Geometry check sheet. Reference: the model listing, model coordinates, mm. Face numbers are marked on the shaded views. A direction names the side the tool comes from. Coordinates: 2 decimals unless noted, no trailing zeros. Loops run counter-clockwise (first coordinate to the right, second up) from the corner with the lowest first, then second, coordinate; pieces in that order, holes last. Notation, with made-up numbers: (-17.5, 76.5) - (8.5, 76.5) arc R24 cw to (8.5, 94.5) - close; hole circle Ø9 at (19.5, 35.25). An arc over 180 degrees is marked (long way). Write item = value, one per line. Start each with the question number.
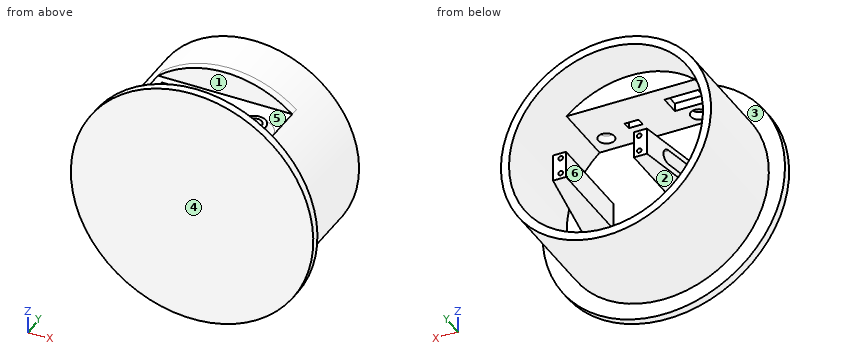
from build123d import *

# Parameters (mm, degrees)
SKETCH4_R                   = 65
SKETCH4_R_2                 = 60
EXTRUDE_THIN1_DEPTH         = 75
SKETCH5_R                   = 75
BOSS_EXTRUDE1_DEPTH         = 5
BOSS_EXTRUDE2_START         = -40
SKETCH6_W                   = 83.06623863
SKETCH6_H                   = 5
BOSS_EXTRUDE2_DEPTH         = 40
CUT_EXTRUDE1_START          = -40
CUT_EXTRUDE1_DEPTH          = 35
SKETCH8_W                   = 7.6
SKETCH8_H                   = 16.75
BOSS_EXTRUDE3_DEPTH         = 57.3
CHAMFER1_SIZE               = 10
CHAMFER1_SIZE_2             = 60
M3_5X0_6_TAPPED_HOLE1_D     = 2.9
M3_5X0_6_TAPPED_HOLE1_DEPTH = 9.128752102
M3_5X0_6_TAPPED_HOLE1_TIP   = 0.871247898
CUT_EXTRUDE2_START          = -57.3
SKETCH11_W                  = 18.622960368
SKETCH11_H                  = 9.279079534
CUT_EXTRUDE2_DEPTH          = 42.3
FILLET1_R                   = 5
CUT_EXTRUDE3_REACH          = 165.936
SKETCH12_R                  = 5.1
SKETCH12_W                  = 20.8
SKETCH12_H                  = 12.6
SKETCH12_W_2                = 8.6
SKETCH12_H_2                = 5
SKETCH13_R                  = 7.5
SKETCH13_R_2                = 5
BOSS_EXTRUDE4_DEPTH         = 5
FILLET2_R                   = 4
CUT_EXTRUDE4_REACH          = 165.936
SKETCH14_R                  = 5


with BuildPart() as part:
    # Sketch4 → Extrude-Thin1 (new body)
    with BuildSketch(Plane(origin=(0, 0, 0), x_dir=(1, 0, 0), z_dir=(0, 1, 0))):
        Circle(SKETCH4_R)
        Circle(SKETCH4_R_2, mode=Mode.SUBTRACT)
    extrude(amount=EXTRUDE_THIN1_DEPTH)

    # Sketch5 → Boss-Extrude1 (add)
    with BuildSketch(Plane(origin=(0, 0, 0), x_dir=(1, 0, 0), z_dir=(0, 1, 0))):
        with Locations(Location((0, 0, 0), (0, 0, 270))):
            Circle(SKETCH5_R)
    extrude(amount=BOSS_EXTRUDE1_DEPTH)

    # Sketch6 → Boss-Extrude2 (add)
    with BuildSketch(Plane(origin=(0, 45, 0), x_dir=(1, 0, 0), z_dir=(0, 1, 0)).offset(BOSS_EXTRUDE2_START)):
        with Locations((0, -47.5)):
            Rectangle(SKETCH6_W, SKETCH6_H)
        with BuildLine():
            Line((41.533119315, -50), (0, -50))
            Line((0, -50), (0, -65))
            ThreePointArc((0, -65), (22.079402166, -61.135096303), (41.533119315, -50))
        make_face()
        with BuildLine():
            Line((0, -65), (0, -50))
            Line((0, -50), (-41.533119315, -50))
            ThreePointArc((-41.533119315, -50), (-22.079402166, -61.135096303), (0, -65))
        make_face()
        with BuildLine():
            Line((41.533119315, -50), (0, -50))
            Line((0, -50), (0, -65))
            ThreePointArc((0, -65), (22.079402166, -61.135096303), (41.533119315, -50))
        make_face()
        with BuildLine():
            Line((0, -65), (0, -50))
            Line((0, -50), (-41.533119315, -50))
            ThreePointArc((-41.533119315, -50), (-22.079402166, -61.135096303), (0, -65))
        make_face()
    extrude(amount=BOSS_EXTRUDE2_DEPTH)

    # Sketch7 → Cut-Extrude1 (cut)
    with BuildSketch(Plane(origin=(0, 45, 0), x_dir=(1, 0, 0), z_dir=(0, 1, 0)).offset(CUT_EXTRUDE1_START)):
        with BuildLine():
            Line((-41.533119315, -50), (41.533119315, -50))
            ThreePointArc((41.533119315, -50), (0, -65), (-41.533119315, -50))
        make_face()
    extrude(amount=CUT_EXTRUDE1_DEPTH, mode=Mode.SUBTRACT)

    # Sketch8 → Boss-Extrude3 (add)
    with BuildSketch(Plane(origin=(0, 5, 0), x_dir=(1, 0, 0), z_dir=(0, 1, 0))):
        with Locations((35, 0.125)):
            Rectangle(SKETCH8_W, SKETCH8_H)
        with Locations((-14.6, 0.125)):
            Rectangle(SKETCH8_W, SKETCH8_H)
    extrude(amount=BOSS_EXTRUDE3_DEPTH)

    # Chamfer1
    # the kernel refuses this chamfer: 60, 10 mm, written as the material it adds along each edge
    with BuildSketch(Plane(origin=(38.8, 5, -8.5), x_dir=(0.9750324932942595, -0.2220622368174739, 0), z_dir=(0, 0, 1))) as chamfer1_piece_1_section:
        Polygon((CHAMFER1_SIZE * 0.975032493294, CHAMFER1_SIZE * 0.222062236817), (-CHAMFER1_SIZE_2 * 0.222062236817, CHAMFER1_SIZE_2 * 0.975032493294), (0, 0), align=None)
    chamfer1_piece_1 = extrude(amount=16.75, mode=Mode.PRIVATE)
    chamfer1_piece_1 = split(chamfer1_piece_1, bisect_by=Plane(origin=(41.528502242, 62.3, -0.125), z_dir=(0, -1, 0)), keep=Keep.TOP, mode=Mode.PRIVATE)
    add(chamfer1_piece_1)
    with BuildSketch(Plane(origin=(-18.4, 5, -8.5), x_dir=(-0.9750324932942595, -0.2220622368174739, 0), z_dir=(0, 0, 1))) as chamfer1_piece_2_section:
        Polygon((CHAMFER1_SIZE * 0.975032493294, -CHAMFER1_SIZE * 0.222062236817), (-CHAMFER1_SIZE_2 * 0.222062236817, -CHAMFER1_SIZE_2 * 0.975032493294), (0, 0), align=None)
    chamfer1_piece_2 = extrude(amount=16.75, mode=Mode.PRIVATE)
    chamfer1_piece_2 = split(chamfer1_piece_2, bisect_by=Plane(origin=(-21.128502242, 62.3, -0.125), z_dir=(0, -1, 0)), keep=Keep.TOP, mode=Mode.PRIVATE)
    add(chamfer1_piece_2)

    # M3.5x0.6 Tapped Hole1
    with Locations(Plane(origin=(0, 62.3, 0), x_dir=(1, 0, 0), z_dir=(0, 1, 0))):
        with Locations((34.5, 4.95), (34.5, -4.95), (-14.1, 4.95), (-14.1, -4.95)):
            Hole(M3_5X0_6_TAPPED_HOLE1_D / 2, depth=M3_5X0_6_TAPPED_HOLE1_DEPTH)
            with Locations((0, 0, -(M3_5X0_6_TAPPED_HOLE1_DEPTH + M3_5X0_6_TAPPED_HOLE1_TIP / 2))):  # 118° drill point
                Cone(0, M3_5X0_6_TAPPED_HOLE1_D / 2, M3_5X0_6_TAPPED_HOLE1_TIP, mode=Mode.SUBTRACT)

    # Sketch11 → Cut-Extrude2 (cut)
    with BuildSketch(Plane(origin=(0, 62.3, 0), x_dir=(1, 0, 0), z_dir=(0, 1, 0)).offset(CUT_EXTRUDE2_START)):
        with Locations((-19.088519816, 0)):
            Rectangle(SKETCH11_W, SKETCH11_H)
    extrude(amount=CUT_EXTRUDE2_DEPTH, mode=Mode.SUBTRACT)

    # Fillet1
    # the kernel refuses this fillet: 5 mm, written as the material it adds along each edge
    with BuildSketch(Plane(origin=(-10.8, 47.3, -4.639539767), x_dir=(0, 0, 1), z_dir=(-1, 0, 0))) as fillet1_piece_1_section:
        with BuildLine():
            CenterArc((FILLET1_R, -FILLET1_R), FILLET1_R, 90, 90)
            Line((0, -FILLET1_R), (0, 0))
            Line((0, 0), (FILLET1_R, 0))
        make_face()
    fillet1_piece_1 = extrude(amount=23.05, mode=Mode.PRIVATE)
    fillet1_piece_1 = split(fillet1_piece_1, bisect_by=Plane(origin=(-21.396510454, 47.020937275, -3.518217567), z_dir=(0.9863939238321439, -0.1643989873053573, 0)), keep=Keep.TOP, mode=Mode.PRIVATE)
    add(fillet1_piece_1)
    with BuildSketch(Plane(origin=(-33.85, 47.3, 4.639539767), x_dir=(0, -1, 0), z_dir=(1, 0, 0))) as fillet1_piece_2_section:
        with BuildLine():
            CenterArc((FILLET1_R, FILLET1_R), FILLET1_R, 180, 90)
            Line((0, FILLET1_R), (0, 0))
            Line((0, 0), (FILLET1_R, 0))
        make_face()
    fillet1_piece_2 = extrude(amount=23.05, mode=Mode.PRIVATE)
    fillet1_piece_2 = split(fillet1_piece_2, bisect_by=Plane(origin=(-21.396510454, 47.020937275, 3.518217567), z_dir=(0.9863939238321439, -0.1643989873053573, 0)), keep=Keep.TOP, mode=Mode.PRIVATE)
    add(fillet1_piece_2)

    # Sketch12 → Cut-Extrude3 (cut, up to next)
    with BuildSketch(Plane.XY.offset(50), mode=Mode.PRIVATE) as cut_extrude3_sk1:
        with Locations((-26.133119315, 13.4)):
            Circle(SKETCH12_R)
    cut_extrude3_tool1 = extrude(cut_extrude3_sk1.sketch, amount=-CUT_EXTRUDE3_REACH, mode=Mode.PRIVATE) & part.part
    # Sketch12 → Cut-Extrude3 (cut, up to next)
    with BuildSketch(Plane.XY.offset(50), mode=Mode.PRIVATE) as cut_extrude3_sk2:
        with Locations((-26.133119315, 28.7)):
            Rectangle(SKETCH12_W, SKETCH12_H)
    cut_extrude3_tool2 = extrude(cut_extrude3_sk2.sketch, amount=-CUT_EXTRUDE3_REACH, mode=Mode.PRIVATE) & part.part
    # Sketch12 → Cut-Extrude3 (cut, up to next)
    with BuildSketch(Plane.XY.offset(50), mode=Mode.PRIVATE) as cut_extrude3_sk3:
        with Locations((10.2, 21.5)):
            Rectangle(SKETCH12_W_2, SKETCH12_H_2)
    cut_extrude3_tool3 = extrude(cut_extrude3_sk3.sketch, amount=-CUT_EXTRUDE3_REACH, mode=Mode.PRIVATE) & part.part
    add(cut_extrude3_tool1.solids().sort_by_distance((-26.133119, 13.4, 50))[0], mode=Mode.SUBTRACT)
    add(cut_extrude3_tool2.solids().sort_by_distance((-26.133119, 28.7, 50))[0], mode=Mode.SUBTRACT)
    add(cut_extrude3_tool3.solids().sort_by_distance((10.2, 21.5, 50))[0], mode=Mode.SUBTRACT)

    # Sketch13 → Boss-Extrude4 (add)
    with BuildSketch(Plane.XY.offset(50)):
        with Locations(Location((30.033119315, 15.715961892, 0), (0, 0, 180))):
            Circle(SKETCH13_R)
        with Locations((30.033119315, 15.715961892)):
            Circle(SKETCH13_R_2, mode=Mode.SUBTRACT)
    extrude(amount=BOSS_EXTRUDE4_DEPTH)

    # Fillet2
    # the kernel refuses this fillet: 4 mm, written as the material it adds along each edge
    with BuildSketch(Plane(origin=(30.033119315, 15.715961892, 50), x_dir=(-1, 0, 0), z_dir=(0, 1, 0))) as fillet2_piece_1:
        with BuildLine():
            CenterArc((7.5 + FILLET2_R, FILLET2_R), FILLET2_R, 180, 90)
            Line((7.5, FILLET2_R), (7.5, 0))
            Line((7.5, 0), (7.5 + FILLET2_R, 0))
        make_face()
    revolve(axis=Axis((30.033119315, 15.715961892, 50), (0, 0, 1)))

    # Sketch14 → Cut-Extrude4 (cut, up to next)
    with BuildSketch(Plane.XY.offset(50), mode=Mode.PRIVATE) as cut_extrude4_sk1:
        with Locations((30.033119315, 15.715961892)):
            Circle(SKETCH14_R)
    cut_extrude4_tool1 = extrude(cut_extrude4_sk1.sketch, amount=-CUT_EXTRUDE4_REACH, mode=Mode.PRIVATE) & part.part
    add(cut_extrude4_tool1.solids().sort_by_distance((30.033119, 15.715962, 50))[0], mode=Mode.SUBTRACT)


solid = part.part
(1) Draft check along Y on the marked faces 5, 6 and 7. Enter one of: pulls with the +Y half, pulls with the -Y half, needs draft (parallel to the pull), parting line crosses it, or undercut.
(2) Sectioned sample at C-C on x = 45. Enter the section's corners in (y, z), plus the area to 3 significant figures.
(3) Scan lines: line 1 (X direction, y = 12.5, z = -0.5); line 2 (X direction, y = 58, z = 4); line 3 (Z direction, x = -14.1, y = 56). Record each from-to range of solid material in increasing order.
(4) Sectioned sample at A-A on x = 0. Enter the section's corners in (y, z), plus the area to 4 significant figures.
(5) Sectioned sample at B-B on z = 30. Enter the section's corners in (x, y), plus the area to 3 significant figures.
(6) Depth check by flat-ended pin: pin 1 (5.5 mm diameter, centred on x = -23.5, y = 27, fed in from -Z); pin 2 (4 mm diameter, centred on y = 48, z = -35.5, fed in from -X); pin 3 (8 mm diameter, centred on y = 54.5, z = -50.5, fed in from +X). Enter the tip coordinate at first touch or a pass-through.
(7) Tool access check on the marked faces 1, 2, 3 and 4. Record the directions out of +Z, -Z, +X, -X, +Y, -Y that give a thin tool (end or side, any length) a straight path to the whole face; none if there is none.
Working result:
q1.face_5 = undercut
q1.face_6 = needs draft
q1.face_7 = pulls with the +Y half
q2.outline = (0, -60) - (5, -60) - (5, -46.9) - (75, -46.9) - (75, -39.69) - (5, -39.69) - (5, -8.5) - (27.8, -8.5) - (27.8, 8.25) - (5, 8.25) - (5, 39.69) - (75, 39.69) - (75, 46.9) - (5, 46.9) - (5, 60) - (0, 60) - close
q2.area = 1,990 mm2
q3.line_1 = -65 to -60, 31.2 to 47.55, 60 to 65
q3.line_2 = -64.88 to -59.87, -19.57 to -15.2, -13 to -10.8, 31.2 to 33.4, 35.6 to 39.97, 59.87 to 64.88
q3.line_3 = -63.45 to -58.32, -8.5 to -6.4, -3.5 to 3.5, 6.4 to 8.25, 58.32 to 63.45
q4.outline = (0, -75) - (5, -75) - (5, -65) - (75, -65) - (75, -60) - (5, -60) - (5, 45) - (45, 45) - (45, 60) - (75, 60) - (75, 65) - (40, 65) - (40, 50) - (5, 50) - (5, 75) - (0, 75) - close
q4.area = 1,525 mm2
q5.outline = (-68.74, 0) - (68.74, 0) - (68.74, 5) - (57.66, 5) - (57.66, 75) - (51.96, 75) - (51.96, 5) - (-51.96, 5) - (-51.96, 75) - (-57.66, 75) - (-57.66, 5) - (-68.74, 5) - close
q5.area = 1,490 mm2
q6.pin_1 = -61.6
q6.pin_2 = -55.7
q6.pin_3 = 45.42
q7.face_1 = +Z, +X, -X
q7.face_2 = +Y
q7.face_3 = none
q7.face_4 = +Z, -Z, +X, -X, -Y
